Read the model definition and answer for the solid it produces. Units are mm, in the model's axes. A direction names the side the tool comes from. Give positions to 0.01 mm unless a question says otherwise; leave off trailing zeros. Order: outer loops, then holes, each group sorted by start corner. A loop starts at its lowest first (then second) coordinate and runs counter-clockwise, first axis right, second up.
Item 1: A cutting plane is placed at B-B (x = -37). Write down the section's boundary in (y, z), plus the area to 3 significant figures.
Item 2: A cutting plane is placed at C-C (y = -1). Write down the section's boundary in (x, z), plus the area to 3 significant figures.
Item 3: Which of the six approach directions +Z, -Z, +X, -X, +Y, -Y give full straight-line access (tool end or side, diameter ignored) to faces 1 (the face through (-39.253, -2, 19)), 2 (the face through (-40.553, 0.5, 18.7)), 3 (the face through (-25, -3, 8))?
Item 4: The mould has two halves that part along Z. Classify faces 4 (the face through (-11.053, -1, 19)), 5 (the face through (-24, -2, 30.956)), 6 (the face through (-39.982, 0.507, 3.057)): +Z half, -Z half, draft (parallel to the pull), parting line (faces both ways), or undercut.
Item 5: Given pin 1 Ø2.5 at (y, z) = (-2.5, 21) entering from +X; pin 2 Ø8.5 at (x, z) = (-24.55, 18.76) entering from -Y, each flat-ended and moving along its own axis, determine where each tip first touches the part or whether it passes through.
Item 6: A cutting plane is placed at A-A (y = -3.5). Write down the section's boundary in (x, z), plus the area to 3 significant figures.
Item 7: A cutting plane is placed at D-D (z = 24). Write down the section's boundary in (x, y), plus the area to 3 significant figures.
Item 8: Find the intervals of material crossed by line 1 along Z through (x, y) = (-37.5, -0.25); line 2 along X through (y, z) = (-2.5, 12); line 3 along X through (y, z) = (0.75, 16), in increasing order.
from build123d import *

# Parameters (mm, degrees)
SKETCH_1_W          = 32
SKETCH_1_H          = 32
EXTRUDE_1_DEPTH     = 1
EXTRUDE_2_DEPTH     = 5
SKETCH_2_W          = 27
SKETCH_2_H          = 14
CUT_EXTRUDE_1_DEPTH = 5
SKETCH_4_R          = 11.747624997
EXTRUDE_3_DEPTH     = 2
SKETCH_5_R          = 4.75
CUT_EXTRUDE_2_DEPTH = 0.5
CUT_EXTRUDE_2_TAPER = 37
SKETCH_6_R          = 3.7
CUT_EXTRUDE_3_DEPTH = 8.5
FILLET_1_R          = 2
SKETCH_7_R          = 1
CUT_EXTRUDE_4_DEPTH = 4
CUT_EXTRUDE_4_TAPER = 2


with BuildPart() as part:
    # 草图1 → 凸台-拉伸1 (new body)
    with BuildSketch(Plane(origin=(0, 0, 0), x_dir=(1, 0, 0), z_dir=(0, 1, 0))):
        with Locations((-24.552631543, -18.455578089)):
            Rectangle(SKETCH_1_W, SKETCH_1_H)
    extrude(amount=EXTRUDE_1_DEPTH)

    # 草图3 → 凸台-拉伸2 (add)
    with BuildSketch(Plane.XZ):
        with BuildLine():
            Line((-9.852631543, 8.255578089), (-9.852631543, 29.255578089))
            ThreePointArc((-9.852631543, 29.255578089), (-10.350550015, 30.457659617), (-11.552631543, 30.955578089))
            Line((-11.552631543, 30.955578089), (-37.552631543, 30.955578089))
            ThreePointArc((-37.552631543, 30.955578089), (-38.754713071, 30.457659617), (-39.252631543, 29.255578089))
            Line((-39.252631543, 29.255578089), (-39.252631543, 8.255578089))
            ThreePointArc((-39.252631543, 8.255578089), (-38.754713071, 7.053496561), (-37.552631543, 6.555578089))
            Line((-37.552631543, 6.555578089), (-11.552631543, 6.555578089))
            ThreePointArc((-11.552631543, 6.555578089), (-10.350550015, 7.053496561), (-9.852631543, 8.255578089))
        make_face()
    extrude(amount=EXTRUDE_2_DEPTH)

    # 草图2 → 切除-拉伸1 (cut)
    with BuildSketch(Plane(origin=(0, 1, 0), x_dir=(1, 0, 0), z_dir=(0, 1, 0))):
        with Locations((-24.552631543, -18.455578089)):
            Rectangle(SKETCH_2_W, SKETCH_2_H)
    extrude(amount=-CUT_EXTRUDE_1_DEPTH, mode=Mode.SUBTRACT)

    # 草图4 → 凸台-拉伸3 (add)
    with BuildSketch(Plane.XZ.offset(5)):
        with Locations((-24.552631543, 18.755578089)):
            Circle(SKETCH_4_R)
    extrude(amount=EXTRUDE_3_DEPTH)

    # 草图5 → 切除-拉伸2 (cut)
    with BuildSketch(Plane.XZ.offset(7)):
        with Locations((-24.552631543, 18.755578089)):
            Circle(SKETCH_5_R)
    extrude(amount=-CUT_EXTRUDE_2_DEPTH, taper=CUT_EXTRUDE_2_TAPER, mode=Mode.SUBTRACT)

    # 草图6 → 切除-拉伸3 (cut, through all)
    with BuildSketch(Plane.XZ.offset(6.5)):
        with Locations((-24.552631543, 18.755578089)):
            Circle(SKETCH_6_R)
    extrude(amount=-CUT_EXTRUDE_3_DEPTH, mode=Mode.SUBTRACT)

    # 圆角1
    fillet_1_edges = [part.edges().sort_by_distance(p)[0] for p in [
        (-40.552631543, 0.5, 2.455578089),
        (-8.552631543, 0.5, 2.455578089),
        (-8.552631543, 0.5, 34.455578089),
        (-40.552631543, 0.5, 34.455578089),
    ]]
    fillet(fillet_1_edges, radius=FILLET_1_R)

    # 草图7 → 切除-拉伸4 (cut)
    with BuildSketch(Plane(origin=(0, 1, 0), x_dir=(1, 0, 0), z_dir=(0, 1, 0))):
        with Locations((-24.552631543, -8.255578089)):
            Circle(SKETCH_7_R)
        with Locations((-12.052631543, -8.255578089)):
            Circle(SKETCH_7_R)
        with Locations((-24.552631543, -29.255578089)):
            Circle(SKETCH_7_R)
        with Locations((-12.052631543, -29.255578089)):
            Circle(SKETCH_7_R)
    extrude(amount=-CUT_EXTRUDE_4_DEPTH, taper=CUT_EXTRUDE_4_TAPER, mode=Mode.SUBTRACT)


solid = part.part
Response values:
1. outline: (-5, 6.56) - (0, 6.56) - (0, 2.46) - (1, 2.46) - (1, 11.46) - (-4, 11.46) - (-4, 25.46) - (1, 25.46) - (1, 34.46) - (0, 34.46) - (0, 30.96) - (-5, 30.96) - close
1. area: 84.0 mm2
2. outline: (-39.25, 8.26) arc R1.7 ccw to (-37.55, 6.56) - (-11.55, 6.56) arc R1.7 ccw to (-9.85, 8.26) - (-9.85, 29.26) arc R1.7 ccw to (-11.55, 30.96) - (-37.55, 30.96) arc R1.7 ccw to (-39.25, 29.26) - close; hole (-38.05, 11.46) - (-11.05, 11.46) - (-11.05, 25.46) - (-38.05, 25.46) - close; hole circle Ø1.86 at (-24.55, 8.26); hole circle Ø1.86 at (-24.55, 29.26); hole circle Ø1.86 at (-12.05, 8.26); hole circle Ø1.86 at (-12.05, 29.26)
2. area: 326 mm2
3. face 1: +Z, -Z, -X, -Y
3. face 2: +Z, -Z, -X, +Y, -Y
3. face 3: +Y
4. face 4: undercut
4. face 5: +Z half
4. face 6: -Z half
5. pin 1: stops at x = -9.85
5. pin 2: stops at y = -6.5
6. outline: (-39.25, 8.26) arc R1.7 ccw to (-37.55, 6.56) - (-11.55, 6.56) arc R1.7 ccw to (-9.85, 8.26) - (-9.85, 29.26) arc R1.7 ccw to (-11.55, 30.96) - (-37.55, 30.96) arc R1.7 ccw to (-39.25, 29.26) - close; hole (-38.05, 11.46) - (-11.05, 11.46) - (-11.05, 25.46) - (-38.05, 25.46) - close
6. area: 337 mm2
7. outline: (-40.55, 0) - (-39.25, 0) - (-39.25, -5) - (-35.06, -5) - (-35.06, -7) - (-14.04, -7) - (-14.04, -5) - (-9.85, -5) - (-9.85, 0) - (-8.55, 0) - (-8.55, 1) - (-11.05, 1) - (-11.05, -4) - (-38.05, -4) - (-38.05, 1) - (-40.55, 1) - close
7. area: 86.0 mm2
8. line 1: z = 6.56 to 11.46, 25.46 to 30.96
8. line 2: x = -39.25 to -38.05, -11.05 to -9.85
8. line 3: x = -40.55 to -38.05, -11.05 to -8.55
